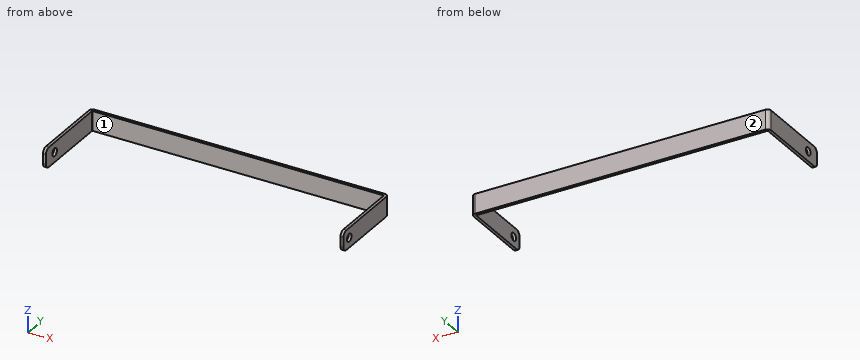
```python
from build123d import *

# Parameters (mm, degrees)
BASE_FLANGE1_DEPTH = 10
SKETCH3_R          = 4
CUT_EXTRUDE1_DEPTH = 307.129466076
FILLET1_R          = 5


# Sheet-metal steps are written as plain solids
with BuildPart() as part:
    # Sketch1 → Base-Flange1 (new, symmetric)
    with BuildSketch(Plane.XY):
        with BuildLine():
            Line((-148.5, -42.5), (-148.5, 36.7634))
            ThreePointArc((-148.5, 36.7634), (-148.284254855, 37.284254855), (-147.7634, 37.5))
            Line((-147.7634, 37.5), (147.7634, 37.5))
            ThreePointArc((147.7634, 37.5), (148.284254855, 37.284254855), (148.5, 36.7634))
            Line((148.5, 36.7634), (148.5, -37.5))
            Line((148.5, -37.5), (151.5, -37.5))
            Line((151.5, -37.5), (151.5, 36.7634))
            ThreePointArc((151.5, 36.7634), (150.405575199, 39.405575199), (147.7634, 40.5))
            Line((147.7634, 40.5), (-147.7634, 40.5))
            ThreePointArc((-147.7634, 40.5), (-150.405575199, 39.405575199), (-151.5, 36.7634))
            Line((-151.5, 36.7634), (-151.5, -42.5))
            Line((-151.5, -42.5), (-148.5, -42.5))
        make_face()
    extrude(amount=BASE_FLANGE1_DEPTH, both=True)

    # Sketch3 → Cut-Extrude1 (cut, through all)
    with BuildSketch(Plane(origin=(151.5, 0, 0), x_dir=(0, 0, -1), z_dir=(1, 0, 0))):
        with Locations(Location((0, -27.5, 0), (0, 0, 90))):
            Circle(SKETCH3_R)
    extrude(amount=-CUT_EXTRUDE1_DEPTH, mode=Mode.SUBTRACT)

    # Fillet1
    fillet1_edges = [part.edges().sort_by_distance(p)[0] for p in [
        (150, -37.5, -10),
        (150, -37.5, 10),
        (-150, -42.5, -10),
        (-150, -42.5, 10),
    ]]
    fillet(fillet1_edges, radius=FILLET1_R)


solid = part.part
```
Source: CAD feature listing. Evaluate the final solid. Frame: model axes, mm. Face numbers are marked on the shaded views. Round coordinates to 2 decimals unless told otherwise and drop trailing zeros. Loops run counter-clockwise (first coordinate to the right, second up) from the corner with the lowest first, then second, coordinate; pieces in that order, holes last.
(1) Material intervals for probe 1 along X at (y, z) = (6, 4.5); probe 2 along Z at (x, y) = (149.15, -27.5); probe 3 along Y at (x, z) = (-51, -1.75), sorted ascending.
From the geometry:
probe 1: x = -151.5 to -148.5, 148.5 to 151.5
probe 2: z = -10 to -4, 4 to 10
probe 3: y = 37.5 to 40.5
(2) Section query C-C (z = 0). Output: boundary loops of the cut face in (x, y), and give its area (3 significant figures).
From the geometry:
outline: (-151.5, -42.5) - (-148.5, -42.5) - (-148.5, -31.5) - (-151.5, -31.5) - close; (-151.5, -23.5) - (-148.5, -23.5) - (-148.5, 36.76) arc R0.74 cw to (-147.76, 37.5) - (147.76, 37.5) arc R0.74 cw to (148.5, 36.76) - (148.5, -23.5) - (151.5, -23.5) - (151.5, 36.76) arc R3.74 ccw to (147.76, 40.5) - (-147.76, 40.5) arc R3.74 ccw to (-151.5, 36.76) - close; (148.5, -37.5) - (151.5, -37.5) - (151.5, -31.5) - (148.5, -31.5) - close
area: 1,320 mm2
(3) Contact query for flat-ended pins moving along their axis: pin 1 Ø6 at (x, z) = (-17, -2.5) entering from -Y; pin 2 Ø3.5 at (x, z) = (150.5, 2.5) entering from -Y; pin 3 Ø6.5 at (y, z) = (-27.5, 0) entering from +X. Output: stop coordinate, or through.
From the geometry:
pin 1: stops at y = 37.5
pin 2: stops at y = -37.5
pin 3: passes through
(4) Section query B-B (y = -27.5). Output: boundary loops of the cut face in (x, z), and give its area (3 significant figures).
From the geometry:
outline: (-151.5, -10) - (-148.5, -10) - (-148.5, -4) - (-151.5, -4) - close; (-151.5, 4) - (-148.5, 4) - (-148.5, 10) - (-151.5, 10) - close; (148.5, -10) - (151.5, -10) - (151.5, -4) - (148.5, -4) - close; (148.5, 4) - (151.5, 4) - (151.5, 10) - (148.5, 10) - close
area: 72.0 mm2
(5) Section query D-D (x = -49). Output: boundary loops of the cut face in (y, z), and give its area (3 significant figures).
From the geometry:
outline: (37.5, -10) - (40.5, -10) - (40.5, 10) - (37.5, 10) - close
area: 60.0 mm2
(6) Pull-direction query (X, two-part tool) for the marked faces 1 and 2; classes: +X half, -X half, draft (parallel to the pull), parting line (faces both ways), or undercut.
From the geometry:
face 1: undercut
face 2: draft
(7) Section query A-A (y = 18). Output: boundary loops of the cut face in (x, z).
From the geometry:
outline: (-151.5, -10) - (-148.5, -10) - (-148.5, 10) - (-151.5, 10) - close; (148.5, -10) - (151.5, -10) - (151.5, 10) - (148.5, 10) - close
